```python
from build123d import *

# Parameters (mm, degrees)
SKETCH1_W           = 88
SKETCH1_H           = 20
SKETCH1_R           = 3.4
BOSS_EXTRUDE1_DEPTH = 7.5
SKETCH2_W           = 10
SKETCH2_H           = 7.5
BOSS_EXTRUDE2_DEPTH = 34
FILLET1_R           = 3


with BuildPart() as part:
    # Sketch1 → Boss-Extrude1 (new body)
    with BuildSketch(Plane.XY):
        with Locations((34, 0)):
            Rectangle(SKETCH1_W, SKETCH1_H)
        Circle(SKETCH1_R, mode=Mode.SUBTRACT)
        with Locations((68, 0)):
            Circle(SKETCH1_R, mode=Mode.SUBTRACT)
    extrude(amount=BOSS_EXTRUDE1_DEPTH)

    # Sketch2 → Boss-Extrude2 (add)
    with BuildSketch(Plane.XZ.offset(10)):
        with Locations((73, 3.75)):
            Rectangle(SKETCH2_W, SKETCH2_H)
    extrude(amount=BOSS_EXTRUDE2_DEPTH)

    # Sketch4 → Loft1 section 0
    with BuildSketch(Plane.XY.offset(7.5)):
        with BuildLine():
            Line((78, -44), (68, -44))
            Line((68, -44), (68, -34))
            Line((68, -34), (78, -34))
            Line((78, -34), (78, -44))
        make_face()
    # Sketch3 → Loft1 section 1
    with BuildSketch(Plane.XY.offset(10.5)):
        with BuildLine():
            Line((75.5, -39), (70.5, -39))
            Line((70.5, -39), (70.5, -44))
            Line((70.5, -44), (75.5, -44))
            Line((75.5, -44), (75.5, -39))
        make_face()
    loft()

    # Fillet1
    fillet1_edges = [part.edges().sort_by_distance(p)[0] for p in [
        (73, -39, 10.5),
        (75.5, -41.5, 10.5),
        (73, -44, 10.5),
        (70.5, -41.5, 10.5),
    ]]
    fillet(fillet1_edges, radius=FILLET1_R - 0.0001)  # a hair under: the kernel refuses the full size


solid = part.part
```
Here's how the part is built. I have some questions about the finished solid (model axes, mm). A direction names the side the tool comes from. Round coordinates to 2 decimals unless told otherwise and drop trailing zeros. Write each loop counter-clockwise with the first axis right and the second up, starting at its lowest first coordinate (ties: lowest second). Pieces come first, ordered by that corner, then holes. Notation, with made-up numbers: M -11,-17.75 L 39,-17.75 A13 ccw 39,5.25 Z; hole C 51,-34.5 d8. An arc over 180 degrees is marked long. Answer as CSV lines item,"result". Start each with the question number.
1. Suppose I cut it at C-C on x = 54.5. Write out the boundary of the cut face in (y, z).
2. Suppose I cut it at A-A on x = 0. Write out the boundary of the cut face in (y, z).
3. Suppose I cut it at D-D on y = -20. Write out the boundary of the cut face in (x, z).
4. Suppose I cut it at B-B on z = 3. Write out the boundary of the cut face in (x, y).
5. On a 3-axis mill with a long thin cutter (end or side, diameter ignored), from which of +Z, -Z, +X, -X, +Y, -Y can I reach the whole of each face in a straight line? I mean faces 5 (the flat face through (33, -2, 7.5)), 6 (the flat face through (68, -27, 4)), 7 (the flat face through (43, -5, 0)). Say none if no direction works.
6. I need wall thicknesses on probe 1 along Y at (x, z) = (0, 2); probe 2 along Z at (x, y) = (54, 7); probe 3 along Y at (x, z) = (49, 7). Which ranges of each line are inside material? Lowest first, please.
7. I'm going to push flat-ended pins straight in: pin 1 Ø2 at (y, z) = (-29.5, 5.5) entering from -X; pin 2 Ø1.5 at (y, z) = (-7.5, 9.5) entering from +X; pin 3 Ø6 at (x, z) = (26.5, 5.5) entering from -Y; pin 4 Ø11 at (x, y) = (68, 0) entering from +Z. Where does each tip first touch, or does it pass through?
8. Thinking about a two-plate mould opening in Y: for faces 1 (the flat face through (73, -44, 4)), 2 (the flat face through (33, 10, 4)), 3 (the cylindrical face through (65.302, -2.069, 3.698)), 4 (the flat face through (-10, 0, 4)), which applies, released by +Y, released by -Y, zero draft, split by the parting line, or undercut?
Check result:
1,outline,"M -10,0 L 10,0 L 10,7.5 L -10,7.5 Z"
2,outline,"M -10,0 L -3.4,0 L -3.4,7.5 L -10,7.5 Z; M 3.4,0 L 10,0 L 10,7.5 L 3.4,7.5 Z"
3,outline,"M 68,0 L 78,0 L 78,7.5 L 68,7.5 Z"
4,outline,"M -10,-10 L 68,-10 L 68,-44 L 78,-44 L 78,10 L -10,10 Z; hole C 0,0 d6.8; hole C 68,0 d6.8"
5,face 5,"+Z, +X, -X, +Y"
5,face 6,"+Z, -Z, -X, -Y"
5,face 7,"-Z, +X, -X, +Y, -Y"
6,probe 1,"y = -10 to -3.4, 3.4 to 10"
6,probe 2,"z = 0 to 7.5"
6,probe 3,"y = -10 to 10"
7,pin 1,"stops at x = 68"
7,pin 2,"passes through"
7,pin 3,"stops at y = -10"
7,pin 4,"stops at z = 7.5"
8,face 1,"released by -Y"
8,face 2,"released by +Y"
8,face 3,"undercut"
8,face 4,"zero draft"
